Read the model definition and answer for the solid it produces. Units are mm, in the model's axes. A direction names the side the tool comes from. Coordinates: 2 decimals unless noted, no trailing zeros. Write each loop counter-clockwise with the first axis right and the second up, starting at its lowest first coordinate (ties: lowest second). Pieces come first, ordered by that corner, then holes. Notation, with made-up numbers: (17, 58.25) -> (43, 58.25) arc R30 cw to (43, 91.25) -> close; hole circle Ø1 at (60, 84.25). An arc over 180 degrees is marked (long way). Write item = value, one per line. Start each with the question number.
1) Flat-ended cylindrical pins translate along their axes: pin 1 Ø3.5 at (x, y) = (-9, 7.5) entering from +Z; pin 2 Ø8 at (y, z) = (12, 59) entering from +X; pin 3 Ø2 at (y, z) = (3.5, 33.5) entering from +X. Find the tip coordinate at first contact, or state that the pin passes through.
2) A tool of negligible diameter and unlimited length cuts with its end or side. For faces 4 (the face through (-6.206, 5.182, 1.479)), 5 (the face through (-8, 8, 3)), from which of +Z, -Z, +X, -X, +Y, -Y can it reach the whole face along a straight path? Write none if from no direction.
3) Find the intervals of material crossed by line 1 along Z through (x, y) = (-14.5, 7.75); line 2 along Y through (x, z) = (-5, 1); line 3 along Y through (x, z) = (-6.25, 20), in increasing order. Write a range as from..to.
4) Section B-B (y = 6.75) is taken. Determine the outline of the cut face in (x, z), plus the area to 3 significant figures.
5) Section D-D (y = 11.25) is taken. Determine the outline of the cut face in (x, z), plus the area to 3 significant figures.
6) Section A-A (x = -5) is taken. Determine the outline of the cut face in (y, z).
7) Section C-C (z = 71) is taken. Determine the outline of the cut face in (x, y).
8) For a pull along Y with two mould halves and no side action, classify faces 1 (the face through (-6, 2, 24)), 2 (the face through (-7.714, 0.798, 44.79)), 3 (the face through (-16.93, 0.6, 45.63)) as released by +Y, released by -Y, zero draft, split by the parting line, or undercut.
Autodesk Inventor part; units mm, degrees
ref_plane "Work Plane1" through (0, 0, 3) normal (0, 0, -1) x (-1, 0, 0)
ref_plane "YZ Plane" through (0, 0, 0) normal (1, 0, 0) x (0, 1, 0)
ref_plane "XZ Plane" through (0, 0, 0) normal (0, 1, 0) x (-1, 0, 0)
sketch "Sketch1" plane through (0, 0, 0) normal (0, 1, 0) x (-1, 0, 0)
  line L0 (0, 0) -> (17.5, 0)
  line L1 (17.5, 0) -> (17.5, 90)
  line L2 (15.5, 90) -> (17.5, 90)
  line L3 (0, 0) -> (15.5, 90)
  dimension "d0" = 90
  dimension "d1" = 17.5
  dimension "d2" = 2
extrude "Extrusion1" add sketch "Sketch1" along normal blind 15
ref_plane "Work Plane1" through (0, 0, 3) normal (0, 0, -1) x (-1, 0, 0)
sketch "Sketch2" plane through (0, 0, 3) normal (0, 0, -1) x (-1, 0, 0)
  line L0 (0, 13) -> (10, 13)
  arc A0 (10, 2) -> (10, 13) centre (10, 7.5) ccw
  line L1 (10, 2) -> (0, 2)
  line L2 (0, 15) -> (0, 13)
  line L3 (0, 2) -> (0, 0)
  line L4 (0, 15) -> (17.5, 15)
  line L5 (0, 0) -> (17.5, 0)
  line L6 (17.5, 15) -> (17.5, 0)
  line L7 (17.5, 0) -> (0, 0)
  line L8 (15.5, 7.5) -> (17.5, 7.5) construction
  line L9 (17.5, 0) -> (17.5, 15) construction
  line L10 (0, 2) -> (0, 13)
  line L11 (0, 0) -> (0, 15)
  dimension "d5" = 2
extrude "Extrusion2" cut sketch "Sketch2" against normal up to surface (87 mm away) contours L0 A0 L1 L10
sketch "Sketch3" plane through (0, 0, 0) normal (0, 0, -1) x (-1, 0, 0)
  circle A0 centre (5, 7.5) radius 2.613
  line L0 (5, 7.5) -> (0, 7.5) construction
  line L1 (0, 0) -> (0, 15)
  dimension "d9" = 5.226
  dimension "d10" = 5
extrude "Extrusion3" cut sketch "Sketch3" against normal blind 10
fillet "Fillet1" radius 2 2 edges at (-17.5, 0, 45) (-17.5, 15, 45)
properties part number "Cable_Chain_Holder"
Answer key:
q1.pin_1 = 3
q1.pin_2 = -9.49
q1.pin_3 = -12.29
q2.face_4 = +Z, -Z
q2.face_5 = +Z, +X
q3.line_1 = 0..3
q3.line_2 = 0..4.89, 10.11..15
q3.line_3 = 0..2, 13..15
q4.outline = (-17.5, 0) -> (-7.5, 0) -> (-7.5, 3) -> (-15.45, 3) -> (-15.45, 89.7) -> (-15.5, 90) -> (-17.5, 90) -> close; (-2.5, 0) -> (0, 0) -> (-0.52, 3) -> (-2.5, 3) -> close
q4.area = 215 mm^2
q5.outline = (-17.5, 0) -> (0, 0) -> (-0.52, 3) -> (-14.02, 3) -> (-14.02, 81.43) -> (-15.5, 90) -> (-17.5, 90) -> close
q5.area = 348 mm^2
q6.outline = (0, 0) -> (4.89, 0) -> (4.89, 3) -> (2, 3) -> (2, 29.03) -> (0, 29.03) -> close; (10.11, 0) -> (15, 0) -> (15, 29.03) -> (13, 29.03) -> (13, 3) -> (10.11, 3) -> close
q7.outline = (-17.5, 2) arc R2 ccw to (-15.5, 0) -> (-12.23, 0) -> (-12.23, 2.47) arc R5.5 cw to (-12.23, 12.53) -> (-12.23, 15) -> (-15.5, 15) arc R2 ccw to (-17.5, 13) -> close
q8.face_1 = undercut
q8.face_2 = zero draft
q8.face_3 = released by -Y
